from build123d import *

# Parameters (mm, degrees)
F0_W     = 4.8
F0_H     = 16.2
F0_H_2   = 19.5
F0_H_3   = 30.6
F0_W_2   = 0.1
F1_DEPTH = 130
F2_DEPTH = 5
F3_SIZE2 = 100
F3_SIZE  = 35
F5_D     = 14.5
F6_DEPTH = 25


with BuildPart() as f1:
    # F0 (on Top) → F1 (new body)
    with BuildSketch(Plane.XY):
        with Locations((2.5, -54.3297186732)):
            Rectangle(F0_W, F0_H)
        with Locations((2.5, -36.4797186732)):
            Rectangle(F0_W, F0_H_2)
        with Locations((2.5, -11.4297186732)):
            Rectangle(F0_W, F0_H_3)
        with Locations((2.5, 13.6202813268)):
            Rectangle(F0_W, F0_H_2)
        with Locations((2.5, 31.4702813268)):
            Rectangle(F0_W, F0_H)
        with Locations((4.95, -36.4797186732)):
            Rectangle(F0_W_2, F0_H_2)
        with Locations((4.95, -54.3297186732)):
            Rectangle(F0_W_2, F0_H)
        with Locations((0.05, -54.3297186732)):
            Rectangle(F0_W_2, F0_H)
        with Locations((0.05, -36.4797186732)):
            Rectangle(F0_W_2, F0_H_2)
        with Locations((0.05, -11.4297186732)):
            Rectangle(F0_W_2, F0_H_3)
        with Locations((4.95, -11.4297186732)):
            Rectangle(F0_W_2, F0_H_3)
        with Locations((4.95, 13.6202813268)):
            Rectangle(F0_W_2, F0_H_2)
        with Locations((0.05, 13.6202813268)):
            Rectangle(F0_W_2, F0_H_2)
        with Locations((0.05, 31.4702813268)):
            Rectangle(F0_W_2, F0_H)
        with Locations((4.95, 31.4702813268)):
            Rectangle(F0_W_2, F0_H)
    extrude(amount=F1_DEPTH)

    # F0 (on Top) → F2 (join)
    with BuildSketch(Plane.XY):
        with Locations((2.5, -36.4797186732)):
            Rectangle(F0_W, F0_H_2)
        with Locations((2.5, 13.6202813268)):
            Rectangle(F0_W, F0_H_2)
    extrude(amount=-F2_DEPTH)

    # F3
    f3_edges = [f1.edges().sort_by_distance(p)[0] for p in [
        (2.5, -62.429719, 130),
        (2.5, 39.570281, 130),
    ]]
    f3_side = f1.faces().sort_by_distance((2.5, -11.429719, 130))[0]
    chamfer(f3_edges, length=F3_SIZE, length2=F3_SIZE2, reference=f3_side)

    # F5 (through all)
    with Locations(Plane.YZ.offset(5)):
        with Locations((-11.4297186732, 75), (-11.3186069886, 110)):
            Hole(F5_D / 2)

    # F4 (on face) → F6 (cut)
    with BuildSketch(Plane.YZ.offset(5)):
        Polygon((-43.0340657718, 70.2807082182), (-39.7305615245, 79.7192917818), (-42.0902074154, 80.5451678437), (-44.4498533063, 81.3710439055), (-47.7533575536, 71.9324603418), align=None)
        Polygon((24.8613753703, 72.0254455898), (21.5602896161, 81.4571191733), (19.2142053056, 80.6359896646), (16.8570168201, 79.803125664), (18.5227448214, 75.0887486929), (20.1884728228, 70.3743717218), align=None)
    extrude(amount=-F6_DEPTH, mode=Mode.SUBTRACT)


solid = f1.part
Can you work these out from the model? Positions are in its coordinate system, mm. A direction names the side the tool comes from. Give positions to 0.01 mm unless a question says otherwise; leave off trailing zeros. Loops run counter-clockwise (first coordinate to the right, second up) from the corner with the lowest first, then second, coordinate; pieces in that order, holes last. Notation, with made-up numbers: (85.5, -1) -> (132.5, -1) arc R20 cw to (132.5, 14) -> close; hole circle Ø4 at (80.25, 37.5). An arc over 180 degrees is marked (long way). Write item = value, one per line.
1) Suppose I cut it at C-C on z = 110. Write out the boundary of the cut face in (x, y), then the cut area to 4 significant figures.
Check result:
outline = (0, -34.43) -> (5, -34.43) -> (5, -18.57) -> (0, -18.57) -> close; (0, -4.07) -> (5, -4.07) -> (5, 11.57) -> (0, 11.57) -> close
area = 157.5 mm2
2) Suppose I cut it at B-B on y = -10. Write out the boundary of the cut face in (x, z).
Check result:
outline = (0, 0) -> (5, 0) -> (5, 67.89) -> (0, 67.89) -> close; (0, 82.11) -> (5, 82.11) -> (5, 102.87) -> (0, 102.87) -> close; (0, 117.13) -> (5, 117.13) -> (5, 130) -> (0, 130) -> close
3) Will these pins go through, and if not, where does the flat tip stop? pin 1 (2.5 mm diameter, centred on x = 2.5, z = -3.5, fed in from +Y); pin 2 (5.5 mm diameter, centred on y = 16, z = -3, fed in from -X); pin 3 (2.5 mm diameter, centred on x = 3.5, z = -1.5, fed in from -Y); pin 4 (8.5 mm diameter, centred on y = -11.43, z = 75, fed in from +X).
Check result:
pin_1 = 23.37
pin_2 = 0.1
pin_3 = -46.23
pin_4 = through
4) Thinking about a two-plate mould opening in Y: for faces 4 (the flat face through (2.535, 22.492, 71.188)), 5 (the flat face through (0, -11, 50)), 6 (the flat face through (2, 23.37, -2)), 7 (the flat face through (2, -11, 0)), which applies, released by +Y, released by -Y, zero draft, split by the parting line, or undercut?
Check result:
face_4 = undercut
face_5 = zero draft
face_6 = released by +Y
face_7 = undercut
5) For faces 1 (the flat face through (2, -26.73, -2)), 2 (the flat face through (2.54, -45.43, 71.12)), 3 (the flat face through (2, -46.23, -2)), which set-ups out of +Z, -Z, +X, -X, +Y, -Y let a thin tool reach every point of the face, with its end or its side?
Check result:
face_1 = -Z, +X, -X
face_2 = +X, -X
face_3 = -Z, +X, -X, -Y
6) Suppose I cut it at D-D on z = 52.5. Write out the boundary of the cut face in (x, y).
Check result:
outline = (0, -54.55) -> (5, -54.55) -> (5, 31.7) -> (0, 31.7) -> close
7) I need wall thicknesses on L1, parallel to Z at x = 3.8, y = -14; L2, parallel to Z at x = 4.2, y = -20.5; L3, parallel to Y at x = 0.9, z = 75.5. Which ranges of each line are inside material? Lowest first, please. Write a range as from..to.
Check result:
L1 = 0..68.22, 81.78..103.26, 116.74..130
L2 = 0..130
L3 = -41.21..-18.66, -4.2..18.38
8) Suppose I cut it at A-A on x = 1.55. Write out the boundary of the cut face in (y, z), then the cut area to 3 significant figures.
Check result:
outline = (-62.43, 0) -> (-46.23, 0) -> (-46.23, -5) -> (-26.73, -5) -> (-26.73, 0) -> (3.87, 0) -> (3.87, -5) -> (23.37, -5) -> (23.37, 0) -> (39.57, 0) -> (39.57, 30) -> (24.86, 72.03) -> (20.19, 70.37) -> (16.86, 79.8) -> (19.21, 80.64) -> (21.56, 81.46) -> (4.57, 130) -> (-27.43, 130) -> (-44.45, 81.37) -> (-39.73, 79.72) -> (-43.03, 70.28) -> (-47.75, 71.93) -> (-62.43, 30) -> close; hole circle Ø14.5 at (-11.43, 75); hole circle Ø14.5 at (-11.32, 110)
area = 9,530 mm2
